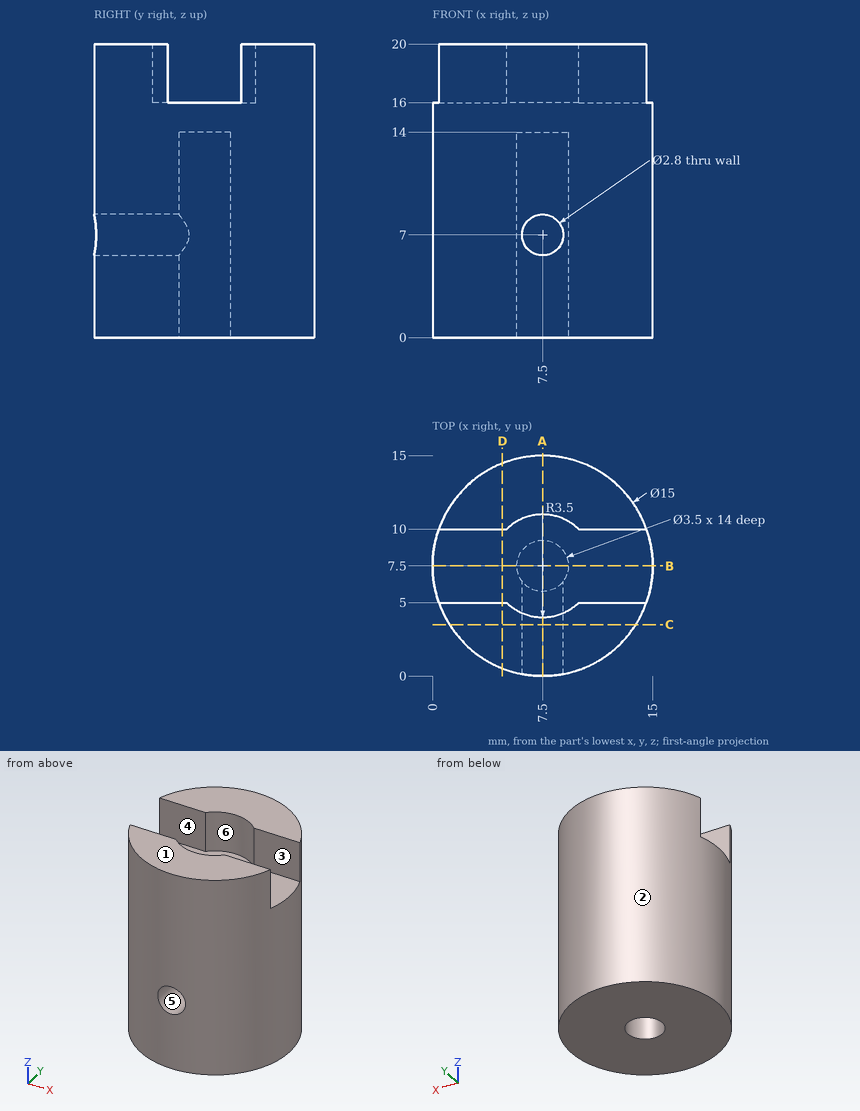
Study the drawing (mm; zero at the part's minimum x, y, z) and answer. A direction names the side the tool comes from. Coordinates: 2 decimals unless noted, no trailing zeros. Loops run counter-clockwise (first coordinate to the right, second up) from the corner with the lowest first, then second, coordinate; pieces in that order, holes last. Notation, with made-up numbers: (57.5, -2.75) -> (87.5, -2.75) arc R17 cw to (87.5, 5.25) -> close; hole circle Ø2 at (56, 19). An arc over 180 degrees is marked (long way). Answer as CSV lines item,"result".
1) For the marked faces 4, 5 and 6, determine the directions among +Z, -Z, +X, -X, +Y, -Y from which every point of the face is accessible in a straight line to the end or side of a thin tool.
A:
face 4,"+Z, +X, -X"
face 5,"-Y"
face 6,"+Z"
2) The part is cut by section C-C (y = 3.5). Give the vertices of the cut face in (x, z).
A:
outline,"(1.16, 0) -> (13.84, 0) -> (13.84, 20) -> (1.16, 20) -> close; hole circle Ø2.8 at (7.5, 7)"
3) The part is cut by section A-A (x = 7.5). Give the vertices of the cut face in (y, z), and give its area (3 significant figures).
A:
outline,"(0, 0) -> (5.75, 0) -> (5.75, 5.6) -> (0, 5.6) -> close; (0, 8.4) -> (5.75, 8.4) -> (5.75, 14) -> (9.25, 14) -> (9.25, 0) -> (15, 0) -> (15, 20) -> (11, 20) -> (11, 16) -> (4, 16) -> (4, 20) -> (0, 20) -> close"
area,"207 mm²"
4) Straight lines are drawn through the part: probe 1 along Y at (x, z) = (5, 2); probe 2 along Z at (x, y) = (3.5, 7); probe 3 along Y at (x, z) = (7.5, 10.5). For each, find the intervals that lie inside material, in ascending order.
A:
probe 1,"y = 0.43 to 14.57"
probe 2,"z = 0 to 16"
probe 3,"y = 0 to 5.75, 9.25 to 15"
5) Flat-ended cylindrical pins translate along their axes: pin 1 (8 mm diameter, centred on x = 10, z = 6, fed in from -Y); pin 2 (4.5 mm diameter, centred on x = 12.5, z = 18.5, fed in from +Y); pin 3 (1.8 mm diameter, centred on x = 7, y = 8, fed in from -Z); pin 4 (2 mm diameter, centred on x = 7.5, y = 7.5, fed in from +Z). Find the tip coordinate at first contact, or state that the pin passes through.
A:
pin 1,"stops at y = 0"
pin 2,"stops at y = 14.48"
pin 3,"stops at z = 14"
pin 4,"stops at z = 16"
6) For a pull along Y with two mould halves and no side action, classify the marked faces 1, 2 and 3 as released by +Y, released by -Y, zero draft, split by the parting line, or undercut.
A:
face 1,"zero draft"
face 2,"split by the parting line"
face 3,"undercut"
7) The part is cut by section B-B (y = 7.5). Give the vertices of the cut face in (x, z).
A:
outline,"(0, 0) -> (5.75, 0) -> (5.75, 14) -> (9.25, 14) -> (9.25, 0) -> (15, 0) -> (15, 16) -> (0, 16) -> close"
8) The part is cut by section D-D (x = 4.75). Give the vertices of the cut face in (y, z), and give its area (3 significant figures).
A:
outline,"(0.52, 0) -> (14.48, 0) -> (14.48, 20) -> (10, 20) -> (10, 16) -> (5, 16) -> (5, 20) -> (0.52, 20) -> close"
area,"259 mm²"
